Read the model definition and answer for the solid it produces. Units are mm, in the model's axes. Face numbers are marked on the shaded views. Give positions to 0.01 mm unless a question says otherwise; leave off trailing zeros. Loops run counter-clockwise (first coordinate to the right, second up) from the corner with the lowest first, then second, coordinate; pieces in that order, holes last. Notation, with made-up numbers: (-1, 50.25) - (23, 50.25) arc R10 ccw to (23, 65.25) - close; hole circle Ø9 at (-31.5, 13). An arc over 180 degrees is marked (long way). Use a Markdown table: item, result. Add a question column.
Item 1: A cutting plane is placed at C-C (z = -5). Determine the outline of the cut face in (x, y).
Item 2: Consider probe 1 along Z at (x, y) = (10, 10.75); probe 2 along X at (y, z) = (5.75, -3.5); probe 3 along Y at (x, z) = (2.75, -8). Determine where each line is inside the solid, lowest interval first. Write a range as [from, to].
Item 3: A cutting plane is placed at D-D (y = 11.5). Determine the outline of the cut face in (x, z).
Item 4: This flat-tipped pin is pushed along its axis until it touches: P1, Ø0.9, axis at x = -10, z = 10, coming from the +Y side. Where does it stop, or does it pass through?
Item 5: A cutting plane is placed at B-B (x = 10). Determine the outline of the cut face in (y, z), plus the area to 3 significant figures.
Item 6: A cutting plane is placed at A-A (y = 7.5). Determine the outline of the cut face in (x, z), plus the area to 3 significant figures.
Item 7: For a pull along X with two mould halves and no side action, classify the marked faces 1, 2, 3 and 4 as +X half, -X half, draft (parallel to the pull), parting line (faces both ways), or undercut.
from build123d import *

# Parameters (mm, degrees)
PAD_DEPTH    = 22.7
SKETCH001_R  = 1.5
POCKET_DEPTH = 3.5


with BuildPart() as part:
    # Sketch → Pad (new body, symmetric)
    with BuildSketch(Plane.XY):
        Polygon((-6, 8), (-6, 3), (-13.5, 3), (-13.5, 13), (13.5, 13), (13.5, 3), (6, 3), (6, 8), align=None)
    extrude(amount=PAD_DEPTH, both=True)

    # Sketch001 → Pocket (cut)
    with BuildSketch(Plane.XZ.offset(-13)):
        with Locations((-10, 10)):
            Circle(SKETCH001_R)
        with Locations((10, 10)):
            Circle(SKETCH001_R)
        with Locations((10, -10)):
            Circle(SKETCH001_R)
        with Locations((-10, -10)):
            Circle(SKETCH001_R)
    extrude(amount=POCKET_DEPTH, mode=Mode.SUBTRACT)


solid = part.part
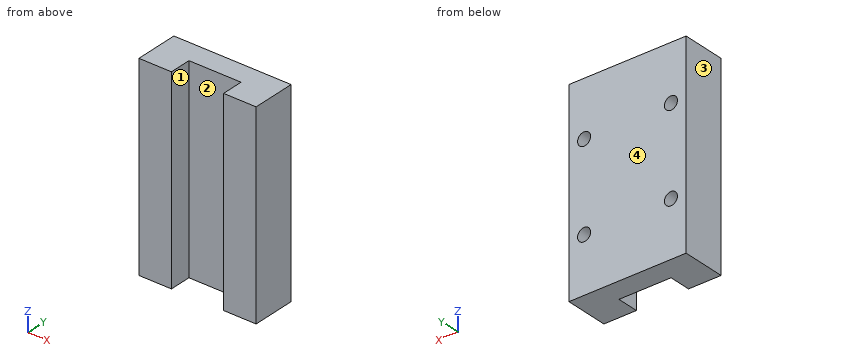
Geometry says:
| question | item | result |
|---|---|---|
| 1 | outline | (-13.5, 3) - (-6, 3) - (-6, 8) - (6, 8) - (6, 3) - (13.5, 3) - (13.5, 13) - (-13.5, 13) - close |
| 2 | probe 1 | [-22.7, -11.5], [-8.5, 8.5], [11.5, 22.7] |
| 2 | probe 2 | [-13.5, -6], [6, 13.5] |
| 2 | probe 3 | [8, 13] |
| 3 | outline | (-13.5, -22.7) - (13.5, -22.7) - (13.5, 22.7) - (-13.5, 22.7) - close; hole circle Ø3 at (-10, -10); hole circle Ø3 at (-10, 10); hole circle Ø3 at (10, -10); hole circle Ø3 at (10, 10) |
| 4 | P1 | y = 9.5 |
| 5 | outline | (3, -22.7) - (13, -22.7) - (13, -11.5) - (9.5, -11.5) - (9.5, -8.5) - (13, -8.5) - (13, 8.5) - (9.5, 8.5) - (9.5, 11.5) - (13, 11.5) - (13, 22.7) - (3, 22.7) - close |
| 5 | area | 433 mm² |
| 6 | outline | (-13.5, -22.7) - (-6, -22.7) - (-6, 22.7) - (-13.5, 22.7) - close; (6, -22.7) - (13.5, -22.7) - (13.5, 22.7) - (6, 22.7) - close |
| 6 | area | 681 mm² |
| 7 | face 1 | undercut |
| 7 | face 2 | undercut |
| 7 | face 3 | -X half |
| 7 | face 4 | draft |
